from build123d import *

# Parameters (mm, degrees)
SKETCH1_R           = 1.6
SKETCH1_R_2         = 2.5
BOSS_EXTRUDE1_DEPTH = 1.57
FILLET1_R           = 5
SKETCH2_R           = 2.5
SKETCH2_R_2         = 1.6
BOSS_EXTRUDE2_DEPTH = 2.93
SKETCH3_R           = 5
SKETCH3_R_2         = 1.6
BOSS_EXTRUDE3_DEPTH = 0.4


with BuildPart() as part:
    # Sketch1 → Boss-Extrude1 (new body)
    with BuildSketch(Plane(origin=(0, 0, 0), x_dir=(1, 0, 0), z_dir=(0, 1, 0))):
        Polygon((-5, -5), (30.925365976, -5), (-5, 23.304833799), align=None)
        with Locations(Location((16.5, 0, 0), (0, 0, 270))):
            Circle(SKETCH1_R, mode=Mode.SUBTRACT)
        with Locations(Location((0, 0, 0), (0, 0, 270))):
            Circle(SKETCH1_R_2, mode=Mode.SUBTRACT)
        with Locations(Location((0, 13, 0), (0, 0, 270))):
            Circle(SKETCH1_R, mode=Mode.SUBTRACT)
    extrude(amount=BOSS_EXTRUDE1_DEPTH)

    # Fillet1
    fillet1_edges = [part.edges().sort_by_distance(p)[0] for p in [
        (-5, 0.785, -23.304833799),
        (30.925365976, 0.785, 5),
        (-5, 0.785, 5),
    ]]
    fillet(fillet1_edges, radius=FILLET1_R)

    # Sketch2 → Boss-Extrude2 (add)
    with BuildSketch(Plane(origin=(0, 1.57, 0), x_dir=(1, 0, 0), z_dir=(0, 1, 0))):
        with BuildLine():
            Line((19.594361133, 3.927458361), (3.094361133, 16.927458361))
            ThreePointArc((3.094361133, 16.927458361), (-2.182681188, 17.498433375), (-5, 13))
            Line((-5, 13), (-5, 0))
            ThreePointArc((-5, 0), (-3.535533906, -3.535533906), (0, -5))
            Line((0, -5), (16.5, -5))
            ThreePointArc((16.5, -5), (21.224261413, -1.637484075), (19.594361133, 3.927458361))
        make_face()
        with Locations(Location((0, 0, 0), (0, 0, 270))):
            Circle(SKETCH2_R, mode=Mode.SUBTRACT)
        with Locations(Location((16.5, 0, 0), (0, 0, 270))):
            Circle(SKETCH2_R_2, mode=Mode.SUBTRACT)
        with Locations(Location((0, 13, 0), (0, 0, 270))):
            Circle(SKETCH2_R_2, mode=Mode.SUBTRACT)
    extrude(amount=BOSS_EXTRUDE2_DEPTH)

    # Sketch3 → Boss-Extrude3 (add)
    # profile 1 of 2: a face of its own
    with BuildSketch(Plane.XZ):
        with Locations(Location((16.5, 0, 0), (0, 0, 270))):
            Circle(SKETCH3_R)
        with Locations(Location((16.5, 0, 0), (0, 0, 270))):
            Circle(SKETCH3_R_2, mode=Mode.SUBTRACT)
    # profile 2 of 2: a face of its own
    with BuildSketch(Plane.XZ):
        with Locations(Location((0, -13, 0), (0, 0, 270))):
            Circle(SKETCH3_R)
        with Locations(Location((0, -13, 0), (0, 0, 270))):
            Circle(SKETCH3_R_2, mode=Mode.SUBTRACT)
    extrude(amount=BOSS_EXTRUDE3_DEPTH)


with BuildPart() as body_2:
    # Mirror1: mirrored copy
    add(part.part.mirror(Plane(origin=(-5, 1.57, -23.304833799), x_dir=(0, 0, 1), z_dir=(1, 0, 0))))


solid = body_2.part
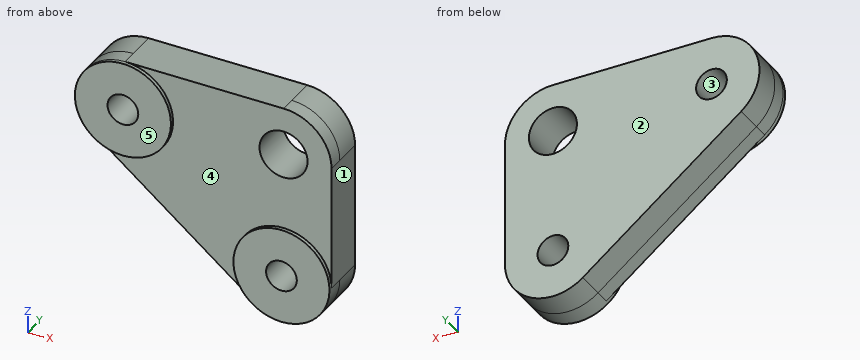
Design review of the part built by this model. Coordinates are the model's own, in mm. Face numbers are marked on the shaded views. A direction names the side the tool comes from. Give positions to 0.01 mm unless a question says otherwise; leave off trailing zeros. Write each loop counter-clockwise with the first axis right and the second up, starting at its lowest first coordinate (ties: lowest second). Pieces come first, ordered by that corner, then holes. Notation, with made-up numbers: M 24.5,86 L 61.5,86 A10 cw 61.5,101 Z; hole C 44.25,15.25 d1. An arc over 180 degrees is marked long. Answer as a JSON object with one key per item and string values. Group by question number.
1) Clearance check with flat-ended pins moving along their axes: pin 1 Ø2.5 at (x, z) = (-10, -13) entering from -Y; pin 2 Ø1 at (x, z) = (-10.5, -5.5) entering from -Y. State where each tip first meets the part, or that it passes through.
2) We need section B-B (z = -12). Give the boundary of the cut face in (x, y).
3) Mouldability with a two-part tool opening along X and no side actions: class the marked faces 1, 2 and 3 as released by +X, released by -X, zero draft, split by the parting line, or undercut.
4) Tool access review of the marked faces 4 and 5: name each direction out of +Z, -Z, +X, -X, +Y, -Y from which nothing blocks a thin tool from reaching the whole face with its end or side.
5) We need section D-D (x = -16.5). Give the boundary of the cut face in (y, z), and give its area (3 significant figures).
6) We need section A-A (y = 2.2). Give the boundary of the cut face in (x, z).
7) We need section C-C (x = -25.75). Give the boundary of the cut face in (y, z).
8) For line 1 along Z through (x, y) = (-10, 3.7); line 2 along X through (y, z) = (1.9, 0); line 3 along Y through (x, z) = (-14.75, -7.25), list the stretches that pass through material, from the lowest coordinate up.
Answer key:
{
 "1": {"pin 1": "passes through", "pin 2": "stops at y = 0"},
 "2": {"outline": "M -19.35,0 L -14.9,0 L -14.9,-0.4 L -11.25,-0.4 L -11.25,4.5 L -19.35,4.5 Z; M -8.75,-0.4 L -5.1,-0.4 L -5.1,0 L -5,0 L -5,4.5 L -8.75,4.5 Z"},
 "3": {"face 1": "released by +X", "face 2": "zero draft", "face 3": "undercut"},
 "4": {"face 4": "-Y", "face 5": "+Z, -Z, +X, -X, -Y"},
 "5": {"outline": "M 0,-14.24 L 4.5,-14.24 L 4.5,5 L 0,5 Z", "area": "86.6 mm²"},
 "6": {"outline": "M -29.59,-3.93 L -13.09,-16.93 A5 ccw -5,-13 L -5,0 A5 ccw -10,5 L -26.5,5 A5 ccw Z; hole C -26.5,0 d3.2; hole C -10,0 d5; hole C -10,-13 d3.2"},
 "7": {"outline": "M -0.4,-4.94 L 0,-4.94 L 0,-6.96 L 4.5,-6.96 L 4.5,-1.41 L -0.4,-1.41 Z; M -0.4,1.41 L 4.5,1.41 L 4.5,5 L 0,5 L 0,4.94 L -0.4,4.94 Z"},
 "8": {"line 1": "z = -18 to -14.6, -11.4 to -2.5, 2.5 to 5", "line 2": "x = -31.5 to -28.1, -24.9 to -12.5, -7.5 to -5", "line 3": "y = 0 to 4.5"}
}
